```python
from build123d import *

# Parameters (mm, degrees)
SKETCH_10_W                   = 100
SKETCH_10_H                   = 110
SM_BASE_FLANGE_2_DEPTH        = 8
SM_EDGE_FLANGE_3_DEPTH        = 100
SM_START                      = 8
SM_EDGE_FLANGE_3_PROFILE_W    = 100
SM_EDGE_FLANGE_3_PROFILE_H    = 106
SM_EDGE_FLANGE_3_PROFILE_R    = 27.5
SM_EDGE_FLANGE_3_FLAT_DEPTH   = 8
SM_EDGE_FLANGE_3_BEND_DEPTH   = 100
SM_EDGE_FLANGE_3_PROFILE_2_W  = 100
SM_EDGE_FLANGE_3_PROFILE_2_H  = 106
SM_EDGE_FLANGE_3_PROFILE_2_R  = 27.5
SM_EDGE_FLANGE_3_FLAT_2_DEPTH = 8
HOLE_WIZARD_M10_1_D           = 8.5
HOLE_WIZARD_M10_1_DEPTH       = 27.5
HOLE_WIZARD_M10_1_TIP         = 2.553657631
FILLET_1_R                    = 50


# Sheet-metal steps are written as plain solids
with BuildPart() as part:
    # 草图10 → 基体-法兰2 (new body)
    with BuildSketch(Plane(origin=(0, 0, 0), x_dir=(1, 0, 0), z_dir=(0, 1, 0))):
        Rectangle(SKETCH_10_W, SKETCH_10_H)
    extrude(amount=-SM_BASE_FLANGE_2_DEPTH)

    # 边线-法兰3 bend section (across the edge) → 边线-法兰3 (add)
    with BuildSketch(Plane(origin=(-50, 0, 63), x_dir=(0, 0, -1), z_dir=(1, 0, 0))):
        with BuildLine():
            Line((-8, 8), (0, 8))
            ThreePointArc((0, 8), (2.343145751, 2.343145751), (8, 0))
            Line((8, 0), (8, -8))
            ThreePointArc((8, -8), (-3.313708499, -3.313708499), (-8, 8))
        make_face()
    extrude(amount=SM_EDGE_FLANGE_3_DEPTH)

    # 边线-法兰3 profile (on flange) → 边线-法兰3 flat (add)
    with BuildSketch(Plane.XY.offset(63).offset(SM_START)):
        with Locations((0, 61)):
            Rectangle(SM_EDGE_FLANGE_3_PROFILE_W, SM_EDGE_FLANGE_3_PROFILE_H)
        with Locations((0, 72)):
            Circle(SM_EDGE_FLANGE_3_PROFILE_R, mode=Mode.SUBTRACT)
    extrude(amount=-SM_EDGE_FLANGE_3_FLAT_DEPTH)

    # 边线-法兰3 bend section 2 (across the edge) → 边线-法兰3 bend (add)
    with BuildSketch(Plane(origin=(50, 0, -63), x_dir=(0, 0, 1), z_dir=(-1, 0, 0))):
        with BuildLine():
            Line((-8, 8), (0, 8))
            ThreePointArc((0, 8), (2.343145751, 2.343145751), (8, 0))
            Line((8, 0), (8, -8))
            ThreePointArc((8, -8), (-3.313708499, -3.313708499), (-8, 8))
        make_face()
    extrude(amount=SM_EDGE_FLANGE_3_BEND_DEPTH)

    # 边线-法兰3 profile 2 (on flange) → 边线-法兰3 flat 2 (add)
    with BuildSketch(Plane(origin=(0, 0, -63), x_dir=(-1, 0, 0), z_dir=(0, 0, -1)).offset(SM_START)):
        with Locations((0, 61)):
            Rectangle(SM_EDGE_FLANGE_3_PROFILE_2_W, SM_EDGE_FLANGE_3_PROFILE_2_H)
        with Locations((0, 72)):
            Circle(SM_EDGE_FLANGE_3_PROFILE_2_R, mode=Mode.SUBTRACT)
    extrude(amount=-SM_EDGE_FLANGE_3_FLAT_2_DEPTH)

    # M10 螺纹孔1
    with Locations(Plane.XY.offset(71)):
        with Locations((30, 20.038475773)):
            Hole(HOLE_WIZARD_M10_1_D / 2, depth=HOLE_WIZARD_M10_1_DEPTH)
            with Locations((0, 0, -(HOLE_WIZARD_M10_1_DEPTH + HOLE_WIZARD_M10_1_TIP / 2))):  # 118° drill point
                Cone(0, HOLE_WIZARD_M10_1_D / 2, HOLE_WIZARD_M10_1_TIP, mode=Mode.SUBTRACT)

    # 圆角1
    fillet_1_edges = [part.edges().sort_by_distance(p)[0] for p in [
        (50, 114, -67),
        (-50, 114, -67),
        (-50, 114, 67),
        (50, 114, 67),
    ]]
    fillet(fillet_1_edges, radius=FILLET_1_R - 0.0001)  # a hair under: the kernel refuses the full size


solid = part.part
```
The listing builds one solid part. Answer for the finished solid, in the listing's coordinates (mm). A direction names the side the tool comes from. Coordinates: 2 decimals unless noted, no trailing zeros. Loops run counter-clockwise (first coordinate to the right, second up) from the corner with the lowest first, then second, coordinate; pieces in that order, holes last. Notation, with made-up numbers: (24, 49.5) -> (47, 49.5) arc R27 ccw to (47, 81.5) -> close; hole circle Ø6 at (28, -22). An arc over 180 degrees is marked (long way). Return JSON: item names as keys, results as strings. Group by question number.
(1) A cutting plane is placed at A-A on y = 47.5. Write down the section's boundary in (x, z), and give its area (3 significant figures).
(2) A cutting plane is placed at D-D on y = 67. Write down the section's boundary in (x, z), and give its area (3 significant figures).
(3) A cutting plane is placed at C-C on x = 30. Write down the section's boundary in (y, z), and give its area (3 significant figures).
(4) Find the intervals of material crossed by probe 1 along Z at (x, y) = (-14, 103); probe 2 along Y at (x, z) = (41.5, 45); probe 3 along Y at (x, z) = (30, 67.25), in increasing order. Write a range as from..to.
(5) A cutting plane is placed at B-B on x = -2. Write down the section's boundary in (y, z).
(6) Given pin 1 Ø12 at (x, z) = (-2.5, -20.5) entering from +Y, flat-ended and moving along its own axis, determine where the tip first touches the part or whether it passes through.
(7) Which of the six approach directions +Z, -Z, +X, -X, +Y, -Y give full straight-line access (tool end or side, diameter ignored) to faces 4 (the cylindrical face through (33.132, 22.911, 66.944)), 5 (the cylindrical face through (35.742, 98.964, -66.944)), 6 (the cylindrical face through (0.7, 2.406, -60.719))?
(8) Determine the mould class of faces 1 (the cylindrical face through (-0.7, -3.437, 66.189)), 2 (the cylindrical face through (3.58, 99.266, -67.056)), 3 (the flat face through (50, -2, -11)) for opening direction Y: released by +Y, released by -Y, zero draft, split by the parting line, or undercut.
The answers:
{
 "1": {"outline": "(-50, -71) -> (-12.49, -71) -> (-12.49, -63) -> (-50, -63) -> close; (-50, 63) -> (-12.49, 63) -> (-12.49, 71) -> (-50, 71) -> close; (12.49, -71) -> (50, -71) -> (50, -63) -> (12.49, -63) -> close; (12.49, 63) -> (50, 63) -> (50, 71) -> (12.49, 71) -> close", "area": "1,200 mm^2"},
 "2": {"outline": "(-49.91, -71) -> (-27.04, -71) -> (-27.04, -63) -> (-49.91, -63) -> close; (-49.91, 63) -> (-27.04, 63) -> (-27.04, 71) -> (-49.91, 71) -> close; (27.04, -71) -> (49.91, -71) -> (49.91, -63) -> (27.04, -63) -> close; (27.04, 63) -> (49.91, 63) -> (49.91, 71) -> (27.04, 71) -> close", "area": "732 mm^2"},
 "3": {"outline": "(-8, -55) arc R16 ccw to (8, -71) -> (104, -71) -> (104, -63) -> (8, -63) arc R8 cw to (0, -55) -> (0, 55) arc R8 cw to (8, 63) -> (15.79, 63) -> (15.79, 71) -> (8, 71) arc R16 ccw to (-8, 55) -> close; (24.29, 63) -> (104, 63) -> (104, 71) -> (24.29, 71) -> close", "area": "2,650 mm^2"},
 "4": {"probe 1": "z = -71..-63, 63..71", "probe 2": "y = -8..0", "probe 3": "y = -2.29..15.79, 24.29..104"},
 "5": {"outline": "(-8, -55) arc R16 ccw to (8, -71) -> (44.57, -71) -> (44.57, -63) -> (8, -63) arc R8 cw to (0, -55) -> (0, 55) arc R8 cw to (8, 63) -> (44.57, 63) -> (44.57, 71) -> (8, 71) arc R16 ccw to (-8, 55) -> close; (99.43, -71) -> (113.96, -71) -> (113.96, -63) -> (99.43, -63) -> close; (99.43, 63) -> (113.96, 63) -> (113.96, 71) -> (99.43, 71) -> close"},
 "6": {"pin 1": "stops at y = 0"},
 "7": {"face 4": "+Z", "face 5": "+Z, -Z, +X, +Y", "face 6": "+X, -X, +Y"},
 "8": {"face 1": "released by -Y", "face 2": "undercut", "face 3": "zero draft"}
}
